```python
from build123d import *

# Parameters (mm, degrees)
F0_R            = 20
F1_DEPTH        = 20
F3_W            = 15
F3_H            = 10
F4_DEPTH        = 30
F4_COPIES_COUNT = 4


# Not quite as in the source:
# - a pattern or mirror of a feature is missing from the dataset's text; its kind, count and spacing are read off the source's solid


with BuildPart() as f1:
    # F0 (on Front) → F1 (new body, symmetric)
    with BuildSketch(Plane.XZ):
        Circle(F0_R)
    extrude(amount=F1_DEPTH, both=True)

    # F3 (on offset) → F4 (join)
    with BuildSketch(Plane.XY.offset(15)):
        Rectangle(F3_W, F3_H)
    f4 = extrude(amount=F4_DEPTH)

    # F4_copies: F4 ×4 about axis
    f4_copies_axis = Axis((0, 0, 0), (0, 1, 0))
    for i in range(1, F4_COPIES_COUNT):
        add(f4.rotate(f4_copies_axis, i * 360 / F4_COPIES_COUNT))


solid = f1.part
```
Part model, mm, in its own coordinate system. A direction names the side the tool comes from. Give positions to 0.01 mm unless a question says otherwise; leave off trailing zeros. Order: outer loops, then holes, each group sorted by start corner. A loop starts at its lowest first (then second) coordinate and runs counter-clockwise, first axis right, second up. Notation, with made-up numbers: (27.25, -4) - (50.25, -4) arc R27 ccw to (50.25, 29) - close; hole circle Ø8 at (-25.5, 72.25). An arc over 180 degrees is marked (long way). Use one line per item in the form item = value.
Item 1: Which spindle directions (+Z, -Z, +X, -X, +Y, -Y) get a long thin tool onto all of the face, cutting with end or side? Do faces 1 (the face through (9.229, -0.28, -17.743)), 2 (the face through (-7.5, 0, 32)), 3 (the face through (-32, 0, -7.5)), 4 (the face through (7.5, 0, 32)). Say none if no direction does.
Solution:
face_1 = none
face_2 = +Z, -X, +Y, -Y
face_3 = -Z, -X, +Y, -Y
face_4 = +Z, +X, +Y, -Y
Item 2: Pin check, flat tips, straight feed: pin 1 Ø1.5 at (x, y) = (16, -10) entering from -Z; pin 2 Ø12 at (y, z) = (-13, -22) entering from +X; pin 3 Ø3 at (y, z) = (-2, -35.5) entering from +X; pin 4 Ø5 at (x, y) = (9, 6.5) entering from -Z. Stop position of each tip, or through.
Solution:
pin_1 = -12.94
pin_2 = 12
pin_3 = 7.5
pin_4 = -45
Item 3: Slice it at C-C on y = 13. Give the cut face in (x, z), and give its area (3 significant figures).
Solution:
outline = circle Ø40 at (0, 0)
area = 1,260 mm2
Item 4: Slice it at B-B on x = 0. Give the cut face in (y, z).
Solution:
outline = (-20, -20) - (-5, -20) - (-5, -45) - (5, -45) - (5, -20) - (20, -20) - (20, 20) - (5, 20) - (5, 45) - (-5, 45) - (-5, 20) - (-20, 20) - close
Item 5: Slice it at D-D on x = -33. Give the cut face in (y, z).
Solution:
outline = (-5, -7.5) - (5, -7.5) - (5, 7.5) - (-5, 7.5) - close
Item 6: Slice it at A-A on z = 0. Give the cut face in (x, y).
Solution:
outline = (-45, -5) - (-20, -5) - (-20, -20) - (20, -20) - (20, -5) - (45, -5) - (45, 5) - (20, 5) - (20, 20) - (-20, 20) - (-20, 5) - (-45, 5) - close
Item 7: Probe probe 1 along X at (y, z) = (3.5, -31); probe 2 along Y at (x, z) = (-1, -28). List the from-to ranges inside material, lowest first. Write a range as from..to.
Solution:
probe_1 = -7.5..7.5
probe_2 = -5..5
